from build123d import *

# Parameters (mm, degrees)
SKETCH1_W           = 68
SKETCH1_H           = 162
BOSS_EXTRUDE1_DEPTH = 12
SKETCH2_W           = 68
SKETCH2_H           = 27
BOSS_EXTRUDE2_DEPTH = 4
SKETCH4_R           = 2.25
CUT_EXTRUDE1_DEPTH  = 171.108788721
SKETCH5_W           = 56.642
SKETCH5_H           = 137.922
CUT_EXTRUDE2_DEPTH  = 3
SKETCH6_W           = 10
SKETCH6_H           = 99
BOSS_EXTRUDE3_DEPTH = 0.746


with BuildPart() as part:
    # Sketch1 → Boss-Extrude1 (new body)
    with BuildSketch(Plane.XY):
        Rectangle(SKETCH1_W, SKETCH1_H)
    extrude(amount=BOSS_EXTRUDE1_DEPTH)

    # Sketch2 → Boss-Extrude2 (add)
    with BuildSketch(Plane(origin=(0, 81, 0), x_dir=(1, 0, 0), z_dir=(0, 1, 0))):
        with Locations((0, 1.5)):
            Rectangle(SKETCH2_W, SKETCH2_H)
    extrude(amount=BOSS_EXTRUDE2_DEPTH)

    # Sketch4 → Cut-Extrude1 (cut, through all)
    with BuildSketch(Plane(origin=(0, 85, 0), x_dir=(1, 0, 0), z_dir=(0, 1, 0))):
        with Locations(Location((0, 10.5, 0), (0, 0, 270))):
            Circle(SKETCH4_R)
    extrude(amount=-CUT_EXTRUDE1_DEPTH, mode=Mode.SUBTRACT)

    # Sketch5 → Cut-Extrude2 (cut)
    with BuildSketch(Plane.XY.offset(12)):
        with Locations((0, -6.039)):
            Rectangle(SKETCH5_W, SKETCH5_H)
    extrude(amount=-CUT_EXTRUDE2_DEPTH, mode=Mode.SUBTRACT)

    # Sketch6 → Boss-Extrude3 (add)
    with BuildSketch(Plane.XY.offset(9)):
        with Locations((0, -25.5)):
            Rectangle(SKETCH6_W, SKETCH6_H)
    extrude(amount=BOSS_EXTRUDE3_DEPTH)


solid = part.part
Source: CAD feature listing. Evaluate the final solid. Frame: model axes, mm. A direction names the side the tool comes from. Coordinates: 2 decimals unless noted, no trailing zeros. Loops run counter-clockwise (first coordinate to the right, second up) from the corner with the lowest first, then second, coordinate; pieces in that order, holes last. Notation, with made-up numbers: (22.5, 30) -> (38.5, 30) arc R12 ccw to (38.5, 49) -> close; hole circle Ø5 at (-4.5, -20.75). An arc over 180 degrees is marked (long way). Answer in a Markdown table with one row per item. Add a question column.
Q1. Section D-D on x = -11. Return the cut outline in (y, z), and give its area (3 significant figures).
Q2. Pull-direction query (Y, two-part tool) for faces 4 (the face through (0, -81, 6)), 5 (the face through (28.321, -7, 11)), 6 (the face through (34, 1, 5)), 7 (the face through (0, 62.922, 11)); classes: pulls with the +Y half, pulls with the -Y half, needs draft (parallel to the pull), parting line crosses it, or undercut.
Q3. Section C-C on y = 58.5. Return the cut outline in (x, z).
Q4. Reachability of faces 1 (the face through (0, -75, 11)), 2 (the face through (0, 1, 0)), 3 (the face through (-0.2, 63.1, 12)) from +Z, -Z, +X, -X, +Y, -Y: full face, straight path, thin tool, end or side. Return the list, or none.
Q5. Ray query, line 1 along X through (y, z) = (84.05, -10.5); line 2 along X through (y, z) = (56, 9.25); line 3 along Y through (x, z) = (10, 9.5). Return the intervals inside material, ascending.
Q6. Contact query for flat-ended pins moving along their axis: pin 1 Ø5 at (x, y) = (-0.5, -2.5) entering from +Z; pin 2 Ø1 at (x, y) = (2, 68) entering from -Z; pin 3 Ø6 at (x, y) = (21.5, -48.5) entering from +Z. Output: stop coordinate, or through.
Q7. Section B-B on x = 0. Return the cut outline in (y, z).
Q8. Section A-A on z = -10.5. Return the cut outline in (x, y).
Computed values:
| question | item | result |
|---|---|---|
| 1 | outline | (-81, 0) -> (81, 0) -> (81, -15) -> (85, -15) -> (85, 12) -> (62.92, 12) -> (62.92, 9) -> (-75, 9) -> (-75, 12) -> (-81, 12) -> close |
| 1 | area | 1,640 mm^2 |
| 2 | face 4 | pulls with the -Y half |
| 2 | face 5 | undercut |
| 2 | face 6 | needs draft |
| 2 | face 7 | undercut |
| 3 | outline | (-34, 0) -> (34, 0) -> (34, 12) -> (28.32, 12) -> (28.32, 9) -> (-28.32, 9) -> (-28.32, 12) -> (-34, 12) -> close |
| 4 | face 1 | +Z |
| 4 | face 2 | -Z, +X, -X, -Y |
| 4 | face 3 | +Z, +X, -X, +Y, -Y |
| 5 | line 1 | x = -34 to -2.25, 2.25 to 34 |
| 5 | line 2 | x = -34 to -28.32, 28.32 to 34 |
| 5 | line 3 | y = -81 to -75, 62.92 to 85 |
| 6 | pin 1 | stops at z = 9.75 |
| 6 | pin 2 | stops at z = 0 |
| 6 | pin 3 | stops at z = 9 |
| 7 | outline | (-81, 0) -> (81, 0) -> (81, -8.25) -> (85, -8.25) -> (85, 12) -> (62.92, 12) -> (62.92, 9) -> (24, 9) -> (24, 9.75) -> (-75, 9.75) -> (-75, 12) -> (-81, 12) -> close; (81, -15) -> (85, -15) -> (85, -12.75) -> (81, -12.75) -> close |
| 8 | outline | (-34, 81) -> (-2.25, 81) -> (-2.25, 85) -> (-34, 85) -> close; (2.25, 81) -> (34, 81) -> (34, 85) -> (2.25, 85) -> close |
